Geometry check sheet. Reference: the model listing, model coordinates, mm. A direction names the side the tool comes from. Coordinates: 2 decimals unless noted, no trailing zeros. Write each loop counter-clockwise with the first axis right and the second up, starting at its lowest first coordinate (ties: lowest second). Pieces come first, ordered by that corner, then holes. Notation, with made-up numbers: (-38.5, 50) -> (11.5, 50) arc R28 cw to (11.5, 81) -> close; hole circle Ø7 at (-17, 70). An arc over 180 degrees is marked (long way). Answer in a Markdown table with one row per item. Add a question column.
1. Cross-section at B-B on z = 0. Give the number of separate pieces and of enclosed holes in the cut face, and give its area (3 significant figures).
2. Cross-section at A-A on x = -35. Record the cut outline in (y, z).
3. Cross-section at D-D on x = -13. Record the cut outline in (y, z), and give its area (3 significant figures).
4. Depth check by flat-ended pin: P1, Ø3, axis at x = 35.5, z = 0.5, coming from the +Y side; P2, Ø5, axis at x = -11, z = 1.5, coming from the -Y side; P3, Ø2, axis at y = 11.5, z = -2.5, coming from the -X side; P4, Ø5, axis at y = 29.5, z = 2, coming from the +X side. Enter the tip coordinate at first touch or a pass-through.
5. Mould release check, pull along X, two halves, no side actions. Record for faces 1 (the flat face through (35.7, 2, 2.3)), 2 (the flat face through (28, 24, 0)), 3 (the flat face through (-30, 25, 0)): pulls with the +X half, pulls with the -X half, needs draft (parallel to the pull), parting line crosses it, or undercut.
6. Set-up check for faces 4 (the flat face through (-35.7, 2, 2.3)), 5 (the flat face through (30, 25, 0)), 6 (the cylindrical face through (28.57, 0.6, 0.07)): record each of +Z, -Z, +X, -X, +Y, -Y from which the full face is reachable in a straight line by a thin tool's end or side.
7. Cross-section at C-C on y = 38.5. Record the cut outline in (x, z), and give its area (3 significant figures).
8. Scan lines: L1, parallel to X at y = 24, z = -0.5; L2, parallel to Z at x = 35, y = 1; L3, parallel to Y at x = 17.5, z = -0.75. Record each from-to range of solid material in increasing order. Write a range as from..to.
```python
from build123d import *

# Parameters (mm, degrees)
F1_DEPTH = 5
F3_D     = 4.4958
F4_R     = 1.99999


# Not quite as in the source:
# - a fillet or chamfer is up to 0.001 mm smaller than in the source, because OpenCascade refuses the exact size


with BuildPart() as f1:
    # F0 (on Top) → F1 (new body, symmetric)
    with BuildSketch(Plane.XY):
        Polygon((0, 47), (0, 45), (28, 45), (28, 0), (40, 0), (40, 2), (30, 2), (30, 47), align=None)
    extrude(amount=F1_DEPTH, both=True)

    # F3 (through all)
    with Locations(Plane(origin=(0, 2, 0), x_dir=(-1, 0, 0), z_dir=(0, 1, 0))):
        with Locations((-35, 0)):
            Hole(F3_D / 2)

    # F4 (radius 2 in the source; OpenCascade refuses exactly that, so slightly less here)
    f4_edges = [f1.edges().sort_by_distance(p)[0] for p in [
        (30, 2, 0),
        (28, 0, 0),
        (40, 2, 0),
    ]]
    fillet(f4_edges, radius=F4_R)

    # F5: F1 across plane


with BuildPart() as f1_1:
    add(f1.part)
    add(f1.part.mirror(Plane.YZ))


solid = f1_1.part
```
Results found:
| question | item | result |
|---|---|---|
| 1 | separate pieces | 3 |
| 1 | enclosed holes | 0 |
| 1 | area | 320 mm^2 |
| 2 | outline | (0, -5) -> (2, -5) -> (2, -2.25) -> (0, -2.25) -> close; (0, 2.25) -> (2, 2.25) -> (2, 5) -> (0, 5) -> close |
| 3 | outline | (45, -5) -> (47, -5) -> (47, 5) -> (45, 5) -> close |
| 3 | area | 20.0 mm^2 |
| 4 | P1 | passes through |
| 4 | P2 | stops at y = 45 |
| 4 | P3 | stops at x = -30 |
| 4 | P4 | stops at x = 30 |
| 5 | face 1 | needs draft |
| 5 | face 2 | undercut |
| 5 | face 3 | pulls with the -X half |
| 6 | face 4 | +Z, -Z, -X, +Y |
| 6 | face 5 | +Z, -Z, +X, +Y |
| 6 | face 6 | +Z, -Z, -Y |
| 7 | outline | (-30, -5) -> (-28, -5) -> (-28, 5) -> (-30, 5) -> close; (28, -5) -> (30, -5) -> (30, 5) -> (28, 5) -> close |
| 7 | area | 40.0 mm^2 |
| 8 | L1 | x = -30..-28, 28..30 |
| 8 | L2 | z = -5..-2.25, 2.25..5 |
| 8 | L3 | y = 45..47 |
